Print and shaded views of the part. All mm, measured from the part's lowest x, y and z. A direction names the side the tool comes from. Give positions to 0.01 mm unless a question says otherwise; leave off trailing zeros. Loops run counter-clockwise (first coordinate to the right, second up) from the corner with the lowest first, then second, coordinate; pieces in that order, holes last.
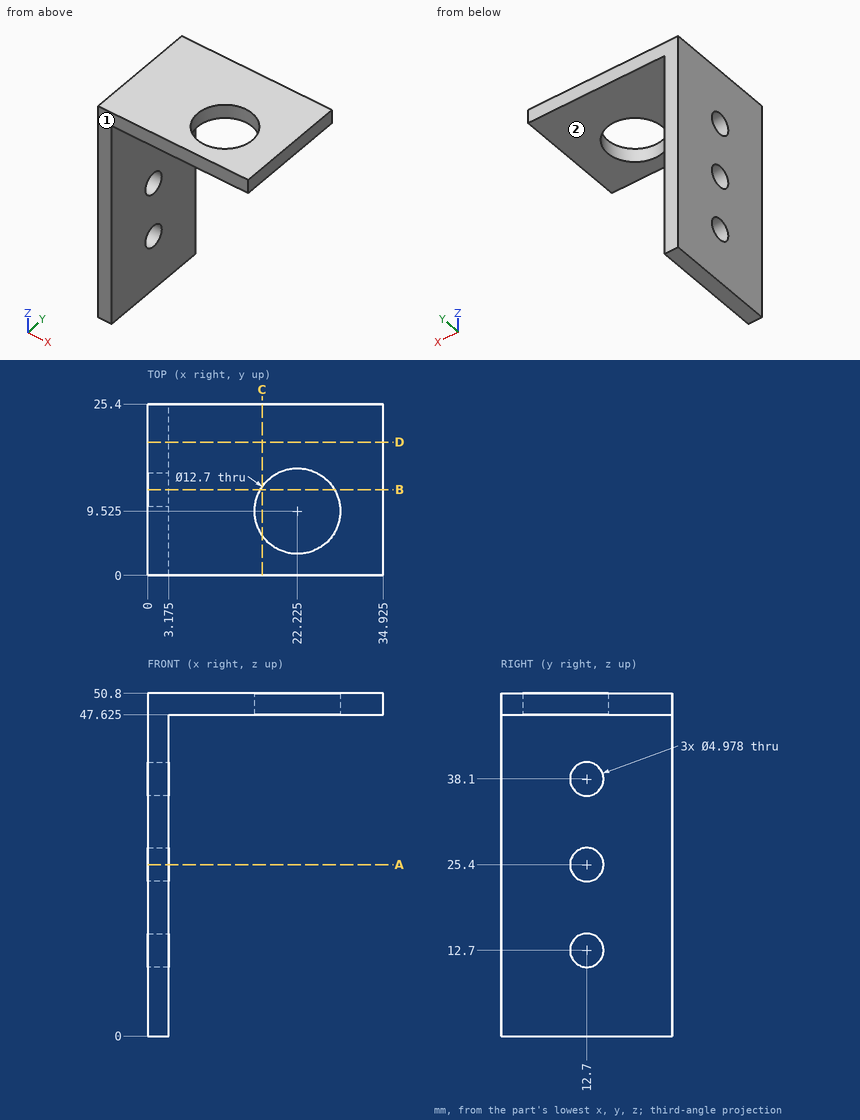
1. Saw through at D-D, the plane y = 19.75. List the corners of the cut face in (x, z) (1 decimal), and give its area (3 significant figures).
Responses:
outline: (0, 0) - (3.2, 0) - (3.2, 47.6) - (34.9, 47.6) - (34.9, 50.8) - (0, 50.8) - close
area: 262 mm2
2. Saw through at C-C, the plane x = 17. List the corners of the cut face in (y, z) (1 decimal).
Responses:
outline: (0, 47.6) - (5.9, 47.6) - (5.9, 50.8) - (0, 50.8) - close; (13.1, 47.6) - (25.4, 47.6) - (25.4, 50.8) - (13.1, 50.8) - close
3. Saw through at B-B, the plane y = 12.7. List the corners of the cut face in (x, z) (1 decimal).
Responses:
outline: (0, 0) - (3.2, 0) - (3.2, 10.2) - (0, 10.2) - close; (0, 15.2) - (3.2, 15.2) - (3.2, 22.9) - (0, 22.9) - close; (0, 27.9) - (3.2, 27.9) - (3.2, 35.6) - (0, 35.6) - close; (0, 40.6) - (3.2, 40.6) - (3.2, 47.6) - (16.7, 47.6) - (16.7, 50.8) - (0, 50.8) - close; (27.7, 47.6) - (34.9, 47.6) - (34.9, 50.8) - (27.7, 50.8) - close
4. Saw through at A-A, the plane z = 25.4. List the corners of the cut face in (x, y) (1 decimal).
Responses:
outline: (0, 0) - (3.2, 0) - (3.2, 10.2) - (0, 10.2) - close; (0, 15.2) - (3.2, 15.2) - (3.2, 25.4) - (0, 25.4) - close
5. Tool access for the marked faces 1 and 2: list every direction of +Z, -Z, +X, -X, +Y, -Y with a clear straight run to the whole face (end or side of a thin tool).
Responses:
face 1: +Z, -Z, +X, -X, -Y
face 2: -Z, +X, +Y, -Y
6. Drop flat-ended pins along their axis: pin 1 (4.5 mm diameter, centred on y = 12.7, z = 12.7, fed in from -X); pin 2 (5 mm diameter, centred on x = 29.5, y = 21, fed in from -Z) (3 decimals); pin 3 (4 mm diameter, centred on y = 13.5, z = 17.5, fed in from +X) (3 decimals). Give the stop position or say it passes through.
Responses:
pin 1: passes through
pin 2: stops at z = 47.625
pin 3: stops at x = 3.175
7. Probe line 1 along Y through (x, z) = (2, 12.7); line 2 along X through (y, z) = (18, 12.5) (1 decimal); line 3 along Z through (x, y) = (14, 16.25) (1 decimal). List the from-to ranges inside material, lowest first.
Responses:
line 1: y = 0 to 10.21, 15.19 to 25.4
line 2: x = 0 to 3.2
line 3: z = 47.6 to 50.8
